The model under review builds one solid part; all positions refer to its coordinate system, in mm. A direction names the side the tool comes from. Round coordinates to 2 decimals unless told otherwise and drop trailing zeros. Loops run counter-clockwise (first coordinate to the right, second up) from the corner with the lowest first, then second, coordinate; pieces in that order, holes last. Notation, with made-up numbers: M 49.5,-3.75 L 75.5,-3.75 A22 ccw 75.5,3.25 Z; hole C 14.5,36.25 d6. An arc over 180 degrees is marked long. Answer as a JSON object with one key per item and string values. Group by question number.
Item 1: Tool access review of faces 5 (the face through (19.2, 18.1, 0)), 6 (the face through (19.05, 29, 3)): name each direction out of +Z, -Z, +X, -X, +Y, -Y from which nothing blocks a thin tool from reaching the whole face with its end or side.
Item 2: To check wall thickness, follow line 1 (Y direction, x = 25.4, z = 3.25); line 2 (Y direction, x = 16, z = 3.75) (3 decimals); line 3 (X direction, y = 27, z = 2.25). State the ranges of each line that lie inside material, in increasing order.
Item 3: Consider section A-A (y = 6.35). Give the boundary of the cut face in (x, z), and give its area (3 significant figures).
Item 4: The part is to be moulded in two halves that separate along X. For faces 1 (the face through (13, 16.669, 3)), 2 (the face through (16, 35.719, 3)), 3 (the face through (0, 18, 3)), 4 (the face through (31.75, 18, 3)), say which applies: +X half, -X half, draft (parallel to the pull), parting line (faces both ways), or undercut.
Item 5: Consider section B-B (x = 25.4). Give the boundary of the cut face in (y, z), and give its area (3 significant figures).
Item 6: Consider section D-D (x = 8). Give the boundary of the cut face in (y, z) (3 decimals).
Item 7: Consider section C-C (z = 1.25). Give the boundary of the cut face in (x, y) (3 decimals).
```python
from build123d import *

# Parameters (mm, degrees)
SKETCH1_R           = 2
SKETCH1_W           = 12.7
SKETCH1_H           = 6.35
BOSS_EXTRUDE1_DEPTH = 6.35


with BuildPart() as part:
    # Sketch1 → Boss-Extrude1 (new body)
    with BuildSketch(Plane.XY):
        Polygon((0, 35.71875), (0, 26.19375), (0, 0), (31.75, 0), (31.75, 26.19375), (31.75, 35.71875), align=None)
        with Locations((25.4, 19.84375)):
            Circle(SKETCH1_R, mode=Mode.SUBTRACT)
        with Locations((25.4, 6.35)):
            Circle(SKETCH1_R, mode=Mode.SUBTRACT)
        with Locations((25.4, 29.36875)):
            Circle(SKETCH1_R, mode=Mode.SUBTRACT)
        with Locations((12.7, 19.84375)):
            Rectangle(SKETCH1_W, SKETCH1_H, mode=Mode.SUBTRACT)
        with Locations((12.7, 6.35)):
            Rectangle(SKETCH1_W, SKETCH1_H, mode=Mode.SUBTRACT)
        with Locations((12.7, 29.36875)):
            Rectangle(SKETCH1_W, SKETCH1_H, mode=Mode.SUBTRACT)
    extrude(amount=BOSS_EXTRUDE1_DEPTH)


solid = part.part
```
Geometry results:
{
 "1": {"face 5": "-Z, +X, -X, +Y, -Y", "face 6": "+Z, -Z"},
 "2": {"line 1": "y = 0 to 4.35, 8.35 to 17.84, 21.84 to 27.37, 31.37 to 35.72", "line 2": "y = 0 to 3.175, 9.525 to 16.669, 23.019 to 26.194, 32.544 to 35.719", "line 3": "x = 0 to 6.35, 19.05 to 31.75"},
 "3": {"outline": "M 0,0 L 6.35,0 L 6.35,6.35 L 0,6.35 Z; M 19.05,0 L 23.4,0 L 23.4,6.35 L 19.05,6.35 Z; M 27.4,0 L 31.75,0 L 31.75,6.35 L 27.4,6.35 Z", "area": "95.6 mm^2"},
 "4": {"face 1": "undercut", "face 2": "draft", "face 3": "-X half", "face 4": "+X half"},
 "5": {"outline": "M 0,0 L 4.35,0 L 4.35,6.35 L 0,6.35 Z; M 8.35,0 L 17.84,0 L 17.84,6.35 L 8.35,6.35 Z; M 21.84,0 L 27.37,0 L 27.37,6.35 L 21.84,6.35 Z; M 31.37,0 L 35.72,0 L 35.72,6.35 L 31.37,6.35 Z", "area": "151 mm^2"},
 "6": {"outline": "M 0,0 L 3.175,0 L 3.175,6.35 L 0,6.35 Z; M 9.525,0 L 16.669,0 L 16.669,6.35 L 9.525,6.35 Z; M 23.019,0 L 26.194,0 L 26.194,6.35 L 23.019,6.35 Z; M 32.544,0 L 35.719,0 L 35.719,6.35 L 32.544,6.35 Z"},
 "7": {"outline": "M 0,0 L 31.75,0 L 31.75,35.719 L 0,35.719 Z; hole M 6.35,3.175 L 19.05,3.175 L 19.05,9.525 L 6.35,9.525 Z; hole M 6.35,16.669 L 19.05,16.669 L 19.05,23.019 L 6.35,23.019 Z; hole M 6.35,26.194 L 19.05,26.194 L 19.05,32.544 L 6.35,32.544 Z; hole C 25.4,6.35 d4; hole C 25.4,19.844 d4; hole C 25.4,29.369 d4"}
}
